The listing builds one solid part. Answer for the finished solid, in the listing's coordinates (mm). Face numbers are marked on the shaded views. Coordinates: 2 decimals unless noted, no trailing zeros. Write each loop counter-clockwise with the first axis right and the second up, starting at its lowest first coordinate (ties: lowest second). Pieces come first, ordered by that corner, then holes.
from build123d import *

# Parameters (mm, degrees)
BOSS_EXTRUDE1_DEPTH = 26.722785591


with BuildPart() as part:
    # Sketch1 → Revolve1 (revolve)
    with BuildSketch(Plane.XY, mode=Mode.PRIVATE) as revolve1_sk:
        Polygon((2, 5.01459854), (2, 21.253819403), (4, 21.253819403), (4, 3.01459854), (7, 3.01459854), (28.722785591, 3.01459854), (28.722785591, 1.01459854), (7, 1.01459854), (2, 1.01459854), align=None)
    revolve(revolve1_sk.sketch.rotate(Axis((2, -2.98540146, 0), (1, 0, 0)), 90), axis=Axis((2, -2.98540146, 0), (1, 0, 0)))

    # Sketch2 → Boss-Extrude1 (add)
    with BuildSketch(Plane.ZY.offset(-2)):
        with BuildLine():
            Line((-0.561713132, -6.945764872), (1.247578239, -6.255500623))
            Line((1.247578239, -6.255500623), (3.056869611, -5.565236374))
            ThreePointArc((3.056869611, -5.565236374), (1.425803702, -6.722657646), (-0.561713132, -6.945764872))
        make_face()
    extrude(amount=-BOSS_EXTRUDE1_DEPTH)


solid = part.part
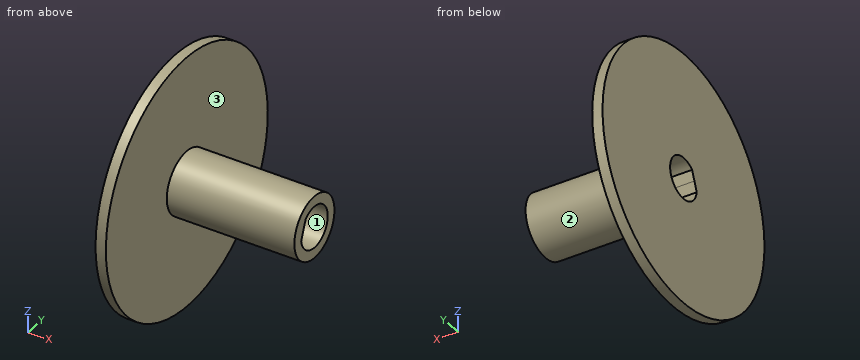
Q1. The part is cut by section B-B, the plane z = -14. Write down the section's boundary in (x, y), then the cut area to 3 significant figures.
Answers below:
outline: (2, -22.77) - (4, -22.77) - (4, 16.8) - (2, 16.8) - close
area: 79.1 mm2
Q2. Given pin 1 (1 mm diameter, centred on y = -11.5, z = 14.5, fed in from +X); pin 2 (6 mm diameter, centred on x = 10.5, y = 0, fed in from -Z); pin 3 (1.5 mm diameter, centred on x = 15.5, y = -5, fed in from -Z), each flat-ended and moving along its own axis, determine where each tip first touches the part or whether it passes through.
Answers below:
pin 1: stops at x = 4
pin 2: stops at z = -6
pin 3: stops at z = -5.87
Q3. Find the intervals of material crossed by probe 1 along X at (y, z) = (11, -6); probe 2 along Y at (x, z) = (19.5, 0); probe 3 along Y at (x, z) = (5.5, 3.5), in increasing order.
Answers below:
probe 1: x = 2 to 4
probe 2: y = -8.99 to -6.73, 1.01 to 3.01
probe 3: y = -7.86 to -4.92, -1.05 to 1.89
Q4. Determine the mould class of the marked faces 1, 2 and 3 for opening direction Z: released by +Z, released by -Z, zero draft, split by the parting line, or undercut.
Answers below:
face 1: undercut
face 2: split by the parting line
face 3: zero draft
Q5. The part is cut by section A-A, the plane x = 26.25. Write down the section's boundary in (y, z), then the cut area to 3 significant figures.
Answers below:
outline: circle Ø12 at (-2.99, 0); hole (-6.95, -0.56) arc R4 ccw (long way) to (-5.57, 3.06) - close
area: 64.1 mm2
Q6. The part is cut by section C-C, the plane y = -14. Write down the section's boundary in (x, z).
Answers below:
outline: (2, -21.59) - (4, -21.59) - (4, 21.59) - (2, 21.59) - close
